Autodesk Inventor part; units mm, degrees
ref_plane "YZ Plane" through (0, 0, 0) normal (1, 0, 0) x (0, 1, 0)
ref_plane "XZ Plane" through (0, 0, 0) normal (0, 1, 0) x (-1, 0, 0)
ref_plane "XY Plane" through (0, 0, 0) normal (0, 0, 1) x (1, 0, 0)
sketch "Sketch1" plane through (0, 0, 0) normal (0, 0, 1) x (1, 0, 0)
  line L0 (-42, -55) -> (42, -55)
  line L1 (42, -55) -> (42, 55)
  line L2 (42, 55) -> (-42, 55)
  line L3 (-42, 55) -> (-42, -55)
  line L4 (-42, -55) -> (42, 55) construction
  line L5 (42, -55) -> (-42, 55) construction
  point P0 (0, 0)
  dimension "d0" = 110
  dimension "d1" = 84
extrude "Extrusion1" add sketch "Sketch1" along normal blind 12
sketch "Sketch2" plane through (0, 0, 12) normal (0, 0, 1) x (1, 0, 0)
  line L0 (0, 80.5745) -> (0, -98.447)
  line L1 (-39.5, 52.5) -> (-39.5, -72.8725)
  line L2 (-39.5, -72.8725) -> (39.5, -72.8725)
  line L3 (39.5, -72.8725) -> (39.5, 52.5)
  line L4 (39.5, 52.5) -> (-39.5, 52.5)
  line L5 (-39.5, 52.5) -> (39.5, -72.8725) construction
  line L6 (-39.5, -72.8725) -> (39.5, 52.5) construction
  line L7 (-42, 55) -> (-42, -55)
  line L8 (42, 55) -> (-42, 55)
  point P0 (0, 0)
  point P1 (0, -10.1862)
  dimension "d4" = 2.5
  dimension "d5" = 2.5
extrude "Extrusion2" cut sketch "Sketch2" against normal blind 7
fillet "Fillet2" radius 2 2 edges at (-39.5, 52.5, 8.5) (39.5, 52.5, 8.5)
fillet "Fillet3" radius 4 2 edges at (-42, 55, 6) (42, 55, 6)
sketch "Sketch4" plane through (0, 0, 5) normal (0, 0, 1) x (1, 0, 0)
  circle A0 centre (-23, -45) radius 5
  line L0 (39.5, -55) -> (-39.5, -55)
  line L1 (0, 77) -> (0, -77)
  point P0 (0, 0)
  dimension "d19" = 10
  dimension "d26" = 23
  dimension "d32" = 10
sketch "Sketch5" plane through (0, 0, 0) normal (1, 0, 0) x (0, 1, 0)
  line L0 (55, 0) -> (55, 12)
  line L1 (55, 7.5) -> (47.2058, 12)
  line L2 (-55, 12) -> (55, 12)
  line L3 (-55, 0) -> (55, 0)
  line L4 (55, 7.5) -> (55, 12)
  line L5 (47.2058, 12) -> (55, 12)
  point P0 (0, 0)
  dimension "d28" = 7.5
  dimension "d29" = 60
sketch "Sketch3" plane through (0, 0, 0) normal (0, 0, -1) x (-1, 0, 0)
  line L0 (-42, -55) -> (-42, 55)
  line L1 (-42, -45) -> (42, -45) construction
  line L2 (42, 55) -> (42, -55)
  line L3 (42, -55) -> (-42, -55)
  point P0 (0, 0)
  point P1 (0, -45)
  point P2 (-23, -45)
  point P3 (23, -45)
  dimension "d8" = 10
  dimension "d10" = 23
  dimension "d11" = 46
sketch "Sketch7" plane through (0, 0, 5) normal (0, 0, 1) x (1, 0, 0)
  line L0 (-42, 55) -> (-42, -55)
  line L1 (-42, 55) -> (-32, 55)
  line L2 (-32, 55) -> (-32, 45)
  line L3 (-32, 45) -> (-42, 45)
  line L4 (-42, 45) -> (-42, 55)
  point P0 (0, 0)
  dimension "d37" = 10
  dimension "d38" = 10
sketch "Sketch8" plane through (0, 0, 5) normal (0, 0, 1) x (1, 0, 0)
  line L0 (-42, 55) -> (-32, 55)
  line L1 (-42, 45) -> (-42, 55)
  line L2 (-42, 55) -> (-42, -55)
  line L3 (-37, 46) -> (-42, 46)
  line L4 (-42, 46) -> (-42, 51)
  line L5 (-42, 51) -> (-37, 51)
  line L6 (-37, 51) -> (-37, 46)
  line L7 (-37, 46) -> (-42, 51) construction
  line L8 (-42, 46) -> (-37, 51) construction
  line L9 (-37, 48.5) -> (-39.5, 48.5) construction
  circle A0 centre (-37, 48.5) radius 2.5
  point P0 (0, 0)
  dimension "d41" = 6.5
  dimension "d42" = 5
  dimension "d43" = 5
properties part number "plate"
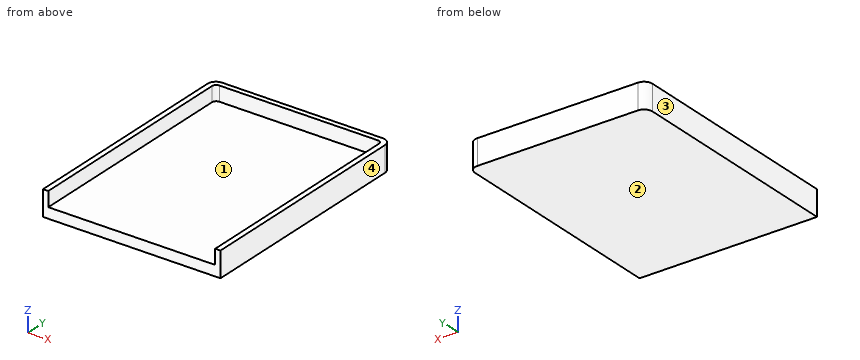
Could you check a few things on this model? Use its own coordinates, in mm. Face numbers are marked on the shaded views. Coordinates: 2 decimals unless noted, no trailing zeros. Write each loop counter-clockwise with the first axis right and the second up, starting at its lowest first coordinate (ties: lowest second). Pieces come first, ordered by that corner, then holes. Notation, with made-up numbers: (-18.5, 75.5) -> (15.5, 75.5) arc R8 cw to (15.5, 79.5) -> close; hole circle Ø2 at (28.5, 22.5). An arc over 180 degrees is marked (long way). Write item = value, one per line. Start each with the question number.
(1) I want a section at A-A (y = -39.5). Please give me the cut outline in (x, z).
(2) I need wall thicknesses on line 1 (X direction, y = -30, z = 7.75); line 2 (Z direction, x = -20, y = -33); line 3 (Y direction, x = -14.5, z = 7.25). Which ranges of each line are inside material? Lowest first, please. Write a range as [from, to].
(3) I want a section at C-C (x = 17.5). Please give me the cut outline in (y, z).
(4) I want a section at B-B (z = 10.5). Please give me the cut outline in (x, y), plus the area to 3 significant figures.
(5) We'd pull the mould along X, two halves only. Please class the marked faces 1, 2, 3 and 4: released by +X, released by -X, zero draft, split by the parting line, or undercut.
(6) Will these pins go through, and if not, where does the flat tip stop? pin 1 (10 mm diameter, centred on x = 16.5, y = 16, fed in from +Z); pin 2 (5.5 mm diameter, centred on x = -2.5, z = 10, fed in from -Y).
Result set:
q1.outline = (-42, 0) -> (42, 0) -> (42, 12) -> (39.5, 12) -> (39.5, 5) -> (-39.5, 5) -> (-39.5, 12) -> (-42, 12) -> close
q2.line_1 = [-42, -39.5], [39.5, 42]
q2.line_2 = [0, 5]
q2.line_3 = [52.5, 55]
q3.outline = (-55, 0) -> (55, 0) -> (55, 12) -> (52.5, 12) -> (52.5, 5) -> (-55, 5) -> close
q4.outline = (-42, -55) -> (-39.5, -55) -> (-39.5, 50.5) arc R2 cw to (-37.5, 52.5) -> (37.5, 52.5) arc R2 cw to (39.5, 50.5) -> (39.5, -55) -> (42, -55) -> (42, 51) arc R4 ccw to (38, 55) -> (-38, 55) arc R4 ccw to (-42, 51) -> close
q4.area = 742 mm2
q5.face_1 = undercut
q5.face_2 = zero draft
q5.face_3 = released by -X
q5.face_4 = released by +X
q6.pin_1 = 5
q6.pin_2 = 52.5
